Check sheet for the drawn part. Datum: minimum x, y, z corner. Units: mm. Give positions to 0.01 mm unless a question says otherwise; leave off trailing zeros. Order: outer loops, then holes, each group sorted by start corner. A loop starts at its lowest first (then second) coordinate and runs counter-clockwise, first axis right, second up. Notation, with made-up numbers: (-12, 3) -> (5, 3) arc R16 ccw to (5, 13) -> close; hole circle Ø4 at (24, 10.5). An arc over 180 degrees is marked (long way). Return JSON: item names as keys, results as strings. Group by question number.
(1) Thickness scan on line 1 along Y through (x, z) = (10.5, 2); line 2 along X through (y, z) = (72.5, 12.75). Record the ranges inside material, lowest first.
(2) Depth check by flat-ended pin: pin 1 Ø4.5 at (x, z) = (46.5, 5.5) entering from -Y; pin 2 Ø0.8 at (x, y) = (77.5, 20) entering from -Z; pin 3 Ø2 at (y, z) = (54, 1.5) entering from +X. Enter the tip coordinate at first touch or a pass-through.
(3) Cross-section at B-B on x = 52. Enter the section's corners in (y, z), then the cut area to 4 significant figures.
(4) Release check for a two-part mould opening along Y. For the marked faces 1 and 2 record: pulls with the +Y half, pulls with the -Y half, needs draft (parallel to the pull), parting line crosses it, or undercut.
(5) Cross-section at A-A on y = 54. State how many separate pieces and enclosed holes the cut face has, then the cut area to 3 significant figures.
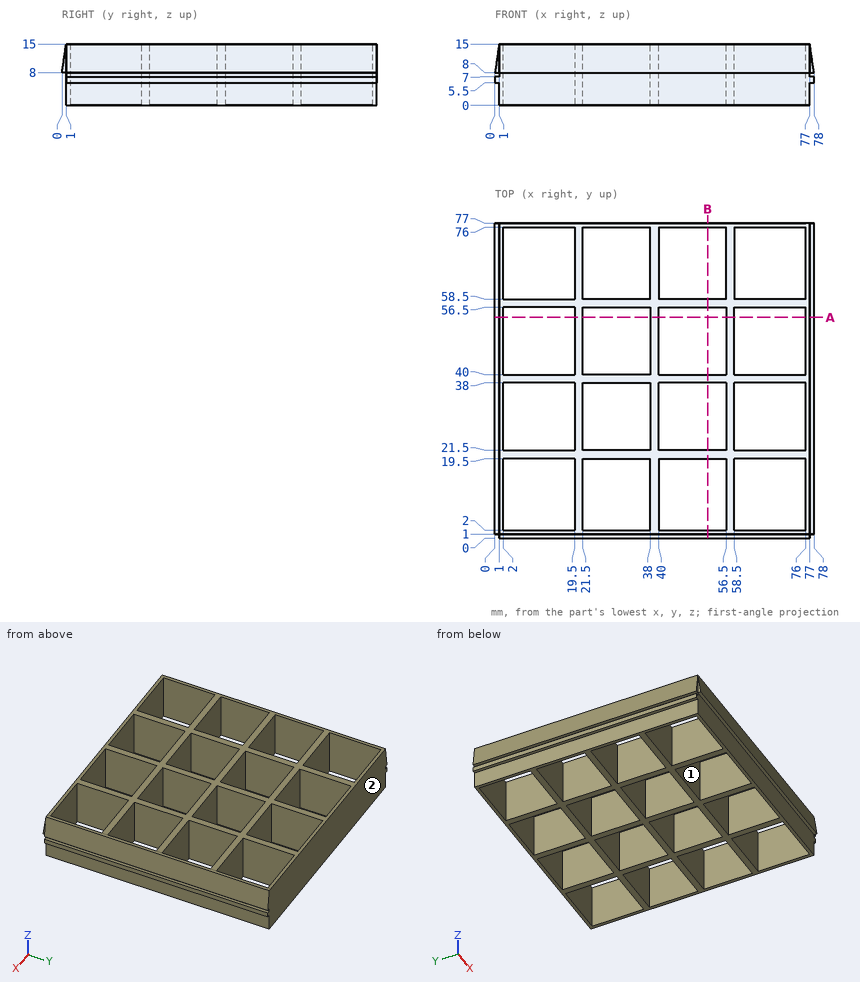
Verdict:
{
 "1": {"line 1": "1 to 2, 19.5 to 21.5, 38 to 40, 56.5 to 58.5, 76 to 77", "line 2": "0.68 to 2, 19.5 to 21.5, 38 to 40, 56.5 to 58.5, 76 to 77.32"},
 "2": {"pin 1": "y = 1", "pin 2": "z = 5.5", "pin 3": "x = 77"},
 "3": {"outline": "(0, 8) -> (1, 8) -> (1, 0) -> (2, 0) -> (2, 15) -> (1, 15) -> close; (19.5, 0) -> (21.5, 0) -> (21.5, 15) -> (19.5, 15) -> close; (38, 0) -> (40, 0) -> (40, 15) -> (38, 15) -> close; (56.5, 0) -> (58.5, 0) -> (58.5, 15) -> (56.5, 15) -> close; (76, 0) -> (77, 0) -> (77, 15) -> (76, 15) -> close", "area": "123.5 mm²"},
 "4": {"face 1": "undercut", "face 2": "pulls with the +Y half"},
 "5": {"separate pieces": "5", "enclosed holes": "0", "area": "130 mm²"}
}
